Could you check a few things on this model? Use its own coordinates, in mm. Face numbers are marked on the shaded views. A direction names the side the tool comes from. Give positions to 0.01 mm unless a question says otherwise; leave off trailing zeros. Order: outer loops, then holes, each group sorted by start corner. A loop starts at its lowest first (then second) coordinate and runs counter-clockwise, first axis right, second up.
(1) Imagine slicing it at A-A, the plane y = 30. Write out the boundary of the cut face in (x, z), then the cut area to 3 significant figures.
(2) Will these pins go through, and if not, where does the flat tip stop? pin 1 (3 mm diameter, centred on x = 22, z = 4, fed in from -Y); pin 2 (4 mm diameter, centred on x = 33, y = 22, fed in from +Z); pin 3 (1.5 mm diameter, centred on x = 10.77, y = 34.71, fed in from -Z).
(3) Imagine slicing it at D-D, the plane y = 21. Write out the boundary of the cut face in (x, z), then the cut area to 3 significant figures.
(4) On a 3-axis mill with a long thin cutter (end or side, diameter ignored), from which of +Z, -Z, +X, -X, +Y, -Y can I reach the whole of each face in a straight line? I mean the marked faces 1 and 2. Say none if no direction works.
(5) If we mould it in two halves opening along X, with no side actions, what happens to the marked faces 3, 4 and 5? For each: released by +X, released by -X, zero draft, split by the parting line, or undercut.
(6) Imagine slicing it at C-C, the plane z = 2.5. State how many separate pieces and enclosed holes the cut face has, then the cut area to 3 significant figures.
(7) If I drill on probe 1 along Y at (x, z) = (10, 2.75); probe 2 along Y at (x, z) = (31, 2.75); probe 3 along X at (y, z) = (30, 2), over which ranges is the centre line in solid material (lowest first)?
(8) Imagine slicing it at B-B, the plane x = 36.5. Write out the boundary of the cut face in (y, z), then the cut area to 3 significant figures.
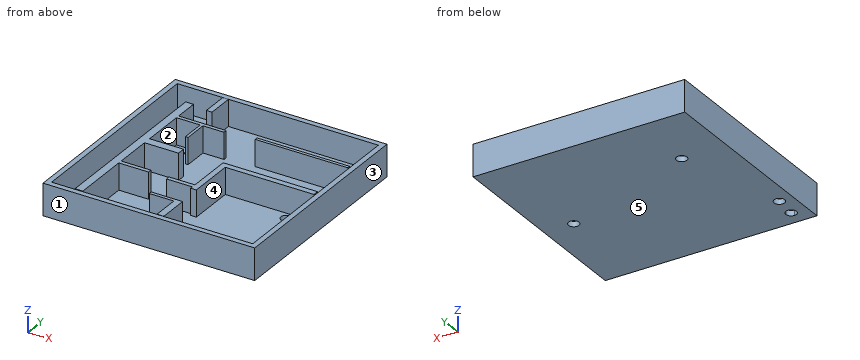
from build123d import *

# Parameters (mm, degrees)
F0_W      = 50.8
F0_H      = 50.8
F1_DEPTH  = 7.62
F2_T      = -1.27
F4_DEPTH  = 25.4
F5_DEPTH  = 6.35
F6_DEPTH  = 25.4
F8_DEPTH  = 6.35
F7_W      = 7.134902291
F7_H      = 0.9276261553
F7_W_2    = 0.6489050575
F7_H_2    = 5.7103633881
F7_R      = 1.27
F7_W_3    = 1.3627009466
F7_H_3    = 6.2943808734
F7_W_4    = 22.2574435174
F7_H_4    = 0.7137954235
F7_W_5    = 21.2840866297
F7_H_5    = 1.362701878
F7_W_6    = 6.2016416341
F7_H_6    = 0.982192345
F7_W_7    = 5.8931484818
F7_H_7    = 0.7639275864
F9_DEPTH  = 6.35
F10_DEPTH = 25.4
F11_DEPTH = 25.4


# Not quite as in the source:
# - a feature names something its author has since deleted; it is built from what else it names


with BuildPart() as f1:
    # F0 (on Top) → F1 (new body)
    with BuildSketch(Plane.XY):
        with Locations((25.4, 25.4)):
            Rectangle(F0_W, F0_H)
    extrude(amount=F1_DEPTH)

    # F2
    f2_openings = [f1.faces().sort_by_distance(p)[0] for p in [
        (25.4, 25.4, 7.62),
    ]]
    offset(amount=F2_T, openings=f2_openings)

    # F3 (on face) → F4 (cut)
    with BuildSketch(Plane.XY.offset(1.27)):
        with BuildLine():
            ThreePointArc((5.08, 3.81), (3.81, 5.08), (2.54, 3.81))
            Line((2.54, 3.81), (3.81, 3.81))
            Line((3.81, 3.81), (3.81, 2.54))
            ThreePointArc((3.81, 2.54), (4.7080256121, 2.9119743879), (5.08, 3.81))
        make_face()
        with BuildLine():
            Line((3.81, 3.81), (2.54, 3.81))
            ThreePointArc((2.54, 3.81), (2.9119743879, 2.9119743879), (3.81, 2.54))
            Line((3.81, 2.54), (3.81, 3.81))
        make_face()
    extrude(amount=-F4_DEPTH, mode=Mode.SUBTRACT)

    # F3 (on face) → F5 (cut)
    with BuildSketch(Plane.XY.offset(1.27)):
        with BuildLine():
            Line((1.27, 49.53), (1.27, 3.81))
            Line((1.27, 3.81), (2.54, 3.81))
            ThreePointArc((2.54, 3.81), (3.81, 5.08), (5.08, 3.81))
            ThreePointArc((5.08, 3.81), (4.7080256121, 2.9119743879), (3.81, 2.54))
            Line((3.81, 2.54), (3.81, 1.27))
            Line((3.81, 1.27), (49.53, 1.27))
            Line((49.53, 1.27), (49.53, 49.53))
            Line((49.53, 49.53), (1.27, 49.53))
        make_face()
    extrude(amount=F5_DEPTH, mode=Mode.SUBTRACT)

    # F3 (on face) → F6 (cut)
    with BuildSketch(Plane.XY.offset(1.27)):
        with BuildLine():
            ThreePointArc((5.08, 3.81), (3.81, 5.08), (2.54, 3.81))
            Line((2.54, 3.81), (3.81, 3.81))
            Line((3.81, 3.81), (3.81, 2.54))
            ThreePointArc((3.81, 2.54), (4.7080256121, 2.9119743879), (5.08, 3.81))
        make_face()
        with BuildLine():
            Line((3.81, 3.81), (2.54, 3.81))
            ThreePointArc((2.54, 3.81), (2.9119743879, 2.9119743879), (3.81, 2.54))
            Line((3.81, 2.54), (3.81, 3.81))
        make_face()
    extrude(amount=-F6_DEPTH, mode=Mode.SUBTRACT)

    # F7 (on face) → F8 (join)
    with BuildSketch(Plane.XY.offset(1.27)):
        Polygon((6.7439782433, 1.4878462534), (8.625802584, 1.4878462534), (8.625802584, 15.2857145295), (8.625802584, 16.2133406848), (8.625802584, 25.1728836447), (8.625802584, 27.1195974201), (8.625802584, 37.4371893704), (8.625802584, 38.2807664573), (8.625802584, 43.9911298454), (6.7439782433, 43.9911298454), align=None)
    extrude(amount=F8_DEPTH)

    # F7 (on face) → F9 (join)
    with BuildSketch(Plane.XY.offset(1.27)):
        Polygon((6.7439782433, 1.4878462534), (8.625802584, 1.4878462534), (8.625802584, 15.2857145295), (8.625802584, 16.2133406848), (8.625802584, 25.1728836447), (8.625802584, 27.1195974201), (8.625802584, 37.4371893704), (8.625802584, 38.2807664573), (8.625802584, 43.9911298454), (6.7439782433, 43.9911298454), align=None)
        with Locations((12.1932537295, 15.7495276071)):
            Rectangle(F7_W, F7_H)
        Polygon((8.625802584, 27.1195974201), (8.625802584, 25.1728836447), (16.8020073324, 25.1728836447), (16.8020073324, 25.9515698999), (16.8020073324, 27.1195974201), align=None)
        Polygon((20.0465321541, 38.2807664573), (8.625802584, 38.2807664573), (8.625802584, 37.4371893704), (14.336167369, 37.4371893704), (14.9850724265, 37.4371893704), (20.0465321541, 37.4371893704), align=None)
        with Locations((14.6606198978, 34.5820076764)):
            Rectangle(F7_W_2, F7_H_2)
        with Locations((10.7671897858, 34.7117893398)):
            Circle(F7_R)
        with Locations((3.3047813922, 9.144927375)):
            Circle(F7_R)
        with Locations((12.8761311062, 46.3596340269)):
            Rectangle(F7_W_3, F7_H_3)
        with Locations((38.118539378, 38.6376641691)):
            Rectangle(F7_W_4, F7_H_4)
        Polygon((27.963174507, 26.6004744917), (26.6004744917, 26.6004744917), (26.6004744917, 15.7768111676), (26.6004744917, 14.7946188226), (26.6004744917, 14.1414962709), (27.963174507, 14.1414962709), (27.963174507, 25.2377726138), align=None)
        with Locations((38.6052178219, 25.9191235527)):
            Rectangle(F7_W_5, F7_H_5)
        with Locations((23.4996536747, 15.2857149951)):
            Rectangle(F7_W_6, F7_H_6)
        with Locations((43.7315702438, 23.4208386391)):
            Circle(F7_R)
        Polygon((28.1472336501, 8.5740732029), (26.510246098, 8.5740732029), (26.510246098, 7.8101456165), (26.510246098, 1.3713347726), (28.1472336501, 1.3713347726), align=None)
        with Locations((23.5636718571, 8.1921094097)):
            Rectangle(F7_W_7, F7_H_7)
    extrude(amount=F9_DEPTH)

    # F10 (cut): faces of the model
    f10_faces = [f1.faces().sort_by_distance(p)[0] for p in [
        (10.7671897858, 34.7117893398, 7.62),
        (3.3047813922, 9.144927375, 7.62),
    ]]
    extrude(f10_faces, amount=-F10_DEPTH, mode=Mode.SUBTRACT)

    # F11 (cut): a face of the model
    f11_faces = [f1.faces().sort_by_distance(p)[0] for p in [
        (43.7315702438, 23.4208386391, 7.62),
    ]]
    extrude(f11_faces, amount=-F11_DEPTH, mode=Mode.SUBTRACT)


solid = f1.part
Answer block:
1. outline: (0, 0) - (50.8, 0) - (50.8, 7.62) - (49.53, 7.62) - (49.53, 1.27) - (8.63, 1.27) - (8.63, 7.62) - (6.74, 7.62) - (6.74, 1.27) - (1.27, 1.27) - (1.27, 7.62) - (0, 7.62) - close
1. area: 92.6 mm2
2. pin 1: stops at y = 0
2. pin 2: stops at z = 1.27
2. pin 3: passes through
3. outline: (0, 0) - (50.8, 0) - (50.8, 7.62) - (49.53, 7.62) - (49.53, 1.27) - (27.96, 1.27) - (27.96, 7.62) - (26.6, 7.62) - (26.6, 1.27) - (8.63, 1.27) - (8.63, 7.62) - (6.74, 7.62) - (6.74, 1.27) - (1.27, 1.27) - (1.27, 7.62) - (0, 7.62) - close
3. area: 101 mm2
4. face 1: +Z, -Z, +X, -X, -Y
4. face 2: +Z
5. face 3: released by +X
5. face 4: undercut
5. face 5: zero draft
6. separate pieces: 6
6. enclosed holes: 1
6. area: 460 mm2
7. probe 1: y = 0 to 1.27, 15.29 to 16.21, 25.17 to 27.12, 37.44 to 38.28, 49.53 to 50.8
7. probe 2: y = 0 to 1.27, 25.24 to 26.6, 38.28 to 38.99, 49.53 to 50.8
7. probe 3: x = 0 to 1.27, 6.74 to 8.63, 49.53 to 50.8
8. outline: (0, 0) - (50.8, 0) - (50.8, 7.62) - (49.53, 7.62) - (49.53, 1.27) - (38.99, 1.27) - (38.99, 7.62) - (38.28, 7.62) - (38.28, 1.27) - (26.6, 1.27) - (26.6, 7.62) - (25.24, 7.62) - (25.24, 1.27) - (1.27, 1.27) - (1.27, 7.62) - (0, 7.62) - close
8. area: 93.8 mm2
